Model file for the job. Use its own axes, mm. A direction names the side the tool comes from. Coordinates: 2 decimals unless noted, no trailing zeros. Write each loop counter-clockwise with the first axis right and the second up, starting at its lowest first coordinate (ties: lowest second). Pieces come first, ordered by that corner, then holes. Notation, with made-up numbers: M 71,-3 L 116,-3 A14 cw 116,6 Z; hole C -5,75 d9. An arc over 180 degrees is marked long. Answer in a Markdown table with one row per item. Add a question column.
Autodesk Fusion 360 part; units mm, degrees
sketch "Esquisse1" plane through (0, 0, 0) normal (0, 0, 1) x (1, 0, 0)
  circle A0 centre (0, 0) radius 8.05
  circle A1 centre (0, 0) radius 4.2
  dimension "d1" = 16.1
  dimension "d2" = 8.4
extrude "Extrusion1" add sketch "Esquisse1" along normal blind 10
sketch "Esquisse2" plane through (0, 0, 0) normal (0, 0, -1) x (1, 0, 0)
  circle A0 centre (0, 0) radius 4.2
  circle A1 centre (0, 0) radius 8.05
  circle A2 centre (0, 0) radius 12.5
  dimension "d5" = 25
extrude "Extrusion2" add sketch "Esquisse2" along normal blind 2 contours A1 | A2
chamfer "Chanfrein1" distance 0.5 angle 45 1 edges at (-7.5052, -2.911, 10)
chamfer "Chanfrein2" distance 0.2 angle 45 1 edges at (-3.9158, -1.5188, -2)
sketch "Esquisse3" plane through (0, 0, -2) normal (0, 0, -1) x (1, 0, 0)
  circle A0 centre (0, 0) radius 12.5
  circle A1 centre (0, 0) radius 4.4
1) Slice it at C-C (z = 8.25). Give the cut face in (x, y), then the cut area to 3 significant figures.
2) Drill centre lines: probe 1 along Y at (x, z) = (0, 4.25); probe 2 along Z at (x, y) = (9.5, -5); probe 3 along X at (y, z) = (-1, 1). Where is each one in solid material? Low to high.
3) Which spindle directions (+Z, -Z, +X, -X, +Y, -Y) get a long thin tool onto all of the face, cutting with end or side? Do faces 1 (the face through (-0.2, 8.2, 0)), 2 (the face through (3.2, -3.2, 10)). Say none if no direction does.
4) Flat gauge pins, fed straight in: pin 1 Ø1 at (x, z) = (-1, -0.5) entering from -Y; pin 2 Ø4 at (y, z) = (7.5, 1.5) entering from -X; pin 3 Ø6 at (y, z) = (4.5, 4.5) entering from -X. Where does each tip first touch, or does it go through?
5) Slice it at D-D (x = -10). Give the cut face in (y, z).
6) Two-plate mould, pull along X, no slides. Class faces 3 (the face through (0, 5, -2)), 4 (the face through (11.923, 3.755, -0.986)), 5 (the face through (4.006, -1.262, 4.017)): released by +X, released by -X, zero draft, split by the parting line, or undercut.
7) Slice it at A-A (y = 0). Give the cut face in (x, z), then the cut area to 3 significant figures.
Ans:
| question | item | result |
|---|---|---|
| 1 | outline | C 0,0 d16.1; hole C 0,0 d8.4 |
| 1 | area | 148 mm2 |
| 2 | probe 1 | y = -8.05 to -4.2, 4.2 to 8.05 |
| 2 | probe 2 | z = -2 to 0 |
| 2 | probe 3 | x = -7.99 to -4.08, 4.08 to 7.99 |
| 3 | face 1 | +Z |
| 3 | face 2 | +Z, +X, -X, +Y, -Y |
| 4 | pin 1 | stops at y = -12.49 |
| 4 | pin 2 | stops at x = -10.87 |
| 4 | pin 3 | stops at x = -7.91 |
| 5 | outline | M -7.5,-2 L 7.5,-2 L 7.5,0 L -7.5,0 Z |
| 6 | face 3 | zero draft |
| 6 | face 4 | split by the parting line |
| 6 | face 5 | undercut |
| 7 | outline | M -12.5,-2 L -4.4,-2 L -4.2,-1.8 L -4.2,10 L -7.55,10 L -8.05,9.5 L -8.05,0 L -12.5,0 Z; M 4.2,-1.8 L 4.4,-2 L 12.5,-2 L 12.5,0 L 8.05,0 L 8.05,9.5 L 7.55,10 L 4.2,10 Z |
| 7 | area | 110 mm2 |
